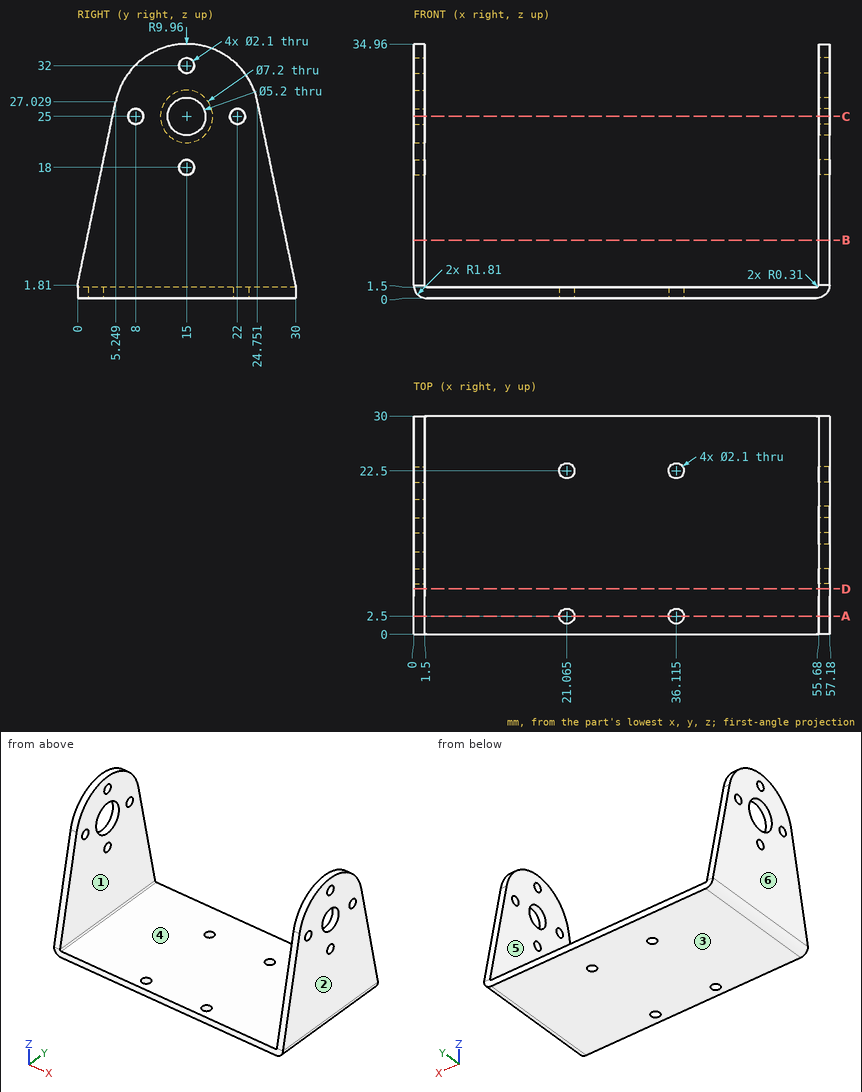
Input: dimensioned drawing with shaded views. Units: mm. Origin: part minimum x, y, z. A direction names the side the tool comes from. Round coordinates to 2 decimals unless told otherwise and drop trailing zeros. Loops run counter-clockwise (first coordinate to the right, second up) from the corner with the lowest first, then second, coordinate; pieces in that order, holes last. Notation, with made-up numbers: (70, 38.5) -> (110, 38.5) arc R13 ccw to (110, 47.5) -> close; hole circle Ø9 at (67.25, -10). An arc over 180 degrees is marked (long way). Use one line per item in the form item = value. Start each with the question number.
1) Section A-A on y = 2.5. Output: boundary loops of the cut face in (x, z) (1 decimal).
2) Section B-B on z = 8. Output: boundary loops of the cut face in (x, y).
3) Access query for the marked faces 5 and 6. Directions: +Z, -Z, +X, -X, +Y, -Y. A direction counts if a zero-diameter tool reaches every point of the face in a straight line with its end or side. Return the directions, or none.
4) Section D-D on y = 6.25. Output: boundary loops of the cut face in (x, z), then the cut area to 3 significant figures.
5) Line query: L1, parallel to X at y = 2.75, z = 5.5; L2, parallel to Z at x = 56.25, y = 15; L3, parallel to Z at x = 46, y = 24. Output: solid intervals per line, ascending.
6) Draft query along X for the marked faces 1, 2, 3 and 4. Return one class per face: released by +X, released by -X, zero draft, split by the parting line, or undercut.
7) First-contact query: P1, Ø4.5, axis at y = 15, z = 25, coming from the -X side; P2, Ø2.5, axis at x = 21.065, y = 22.5, coming from the +Z side. Flat tips, straight axial feed; report the tip coordinate or a pass-through.
8) Section C-C on z = 25. Give the number of separate pieces and of enclosed holes in the cut face.
Response:
q1.outline = (0, 1.8) arc R1.8 ccw to (1.8, 0) -> (20, 0) -> (20, 1.5) -> (1.8, 1.5) arc R0.3 cw to (1.5, 1.8) -> (1.5, 13.8) -> (0, 13.8) -> close; (22.1, 0) -> (35.1, 0) -> (35.1, 1.5) -> (22.1, 1.5) -> close; (37.2, 0) -> (55.4, 0) arc R1.8 ccw to (57.2, 1.8) -> (57.2, 13.8) -> (55.7, 13.8) -> (55.7, 1.8) arc R0.3 cw to (55.4, 1.5) -> (37.2, 1.5) -> close
q2.outline = (0, 1.29) -> (1.5, 1.29) -> (1.5, 28.71) -> (0, 28.71) -> close; (55.68, 1.29) -> (57.18, 1.29) -> (57.18, 28.71) -> (55.68, 28.71) -> close
q3.face_5 = +Z, +Y, -Y
q3.face_6 = +Z, -Z, -X, +Y, -Y
q4.outline = (0, 1.81) arc R1.81 ccw to (1.81, 0) -> (55.37, 0) arc R1.81 ccw to (57.18, 1.81) -> (57.18, 29.76) -> (55.68, 29.76) -> (55.68, 1.81) arc R0.31 cw to (55.37, 1.5) -> (1.81, 1.5) arc R0.31 cw to (1.5, 1.81) -> (1.5, 29.76) -> (0, 29.76) -> close
q4.area = 169 mm^2
q5.L1 = 0 to 1.5, 55.68 to 57.18
q5.L2 = 0.23 to 16.95, 19.05 to 22.4, 27.6 to 30.95, 33.05 to 34.96
q5.L3 = 0 to 1.5
q6.face_1 = undercut
q6.face_2 = released by +X
q6.face_3 = zero draft
q6.face_4 = undercut
q7.P1 = through
q7.P2 = 1.5
q8.separate_pieces = 8
q8.enclosed_holes = 0
